Geometry: final body of the model. Coordinates: model frame, mm. Face numbers are marked on the shaded views. Coordinates: 2 decimals unless noted, no trailing zeros. Loops run counter-clockwise (first coordinate to the right, second up) from the corner with the lowest first, then second, coordinate; pieces in that order, holes last. Notation, with made-up numbers: (11.25, 23) - (62.25, 23) arc R24 cw to (62.25, 51) - close; hole circle Ø10 at (34.5, 69). An arc over 180 degrees is marked (long way). Answer in a Markdown table with one row per item.
from build123d import *

# Parameters (mm, degrees)
SKETCH1_R           = 1.3335
SKETCH1_R_2         = 1.5875
BOSS_EXTRUDE1_DEPTH = 1.651
CHAMFER1_SIZE       = 2.54
SKETCH1_2_R         = 1.5875
BOSS_EXTRUDE2_DEPTH = 2.413
SKETCH1_3_R         = 1.5875
CUT_EXTRUDE1_DEPTH  = 0.889
CUT_EXTRUDE2_DEPTH  = 23.382376376


with BuildPart() as part:
    # Sketch1 → Boss-Extrude1 (new body)
    with BuildSketch(Plane(origin=(0, 0, 0), x_dir=(1, 0, 0), z_dir=(0, 1, 0))):
        with BuildLine():
            Line((-5.567119422, 8.9535), (5.567119422, 8.9535))
            ThreePointArc((5.567119422, 8.9535), (6.35, 6.5405), (7.132880578, 8.9535))
            Line((7.132880578, 8.9535), (20.447, 8.9535))
            Line((20.447, 8.9535), (20.447, -8.9535))
            Line((20.447, -8.9535), (7.132880578, -8.9535))
            ThreePointArc((7.132880578, -8.9535), (6.35, -6.5405), (5.567119422, -8.9535))
            Line((5.567119422, -8.9535), (-5.567119422, -8.9535))
            ThreePointArc((-5.567119422, -8.9535), (-6.35, -6.5405), (-7.132880578, -8.9535))
            Line((-7.132880578, -8.9535), (-20.447, -8.9535))
            Line((-20.447, -8.9535), (-20.447, 8.9535))
            Line((-20.447, 8.9535), (-7.132880578, 8.9535))
            ThreePointArc((-7.132880578, 8.9535), (-6.35, 6.5405), (-5.567119422, 8.9535))
        make_face()
        with Locations(Location((-17.8308, 5.6769, 0), (0, 0, 90))):
            Circle(SKETCH1_R, mode=Mode.SUBTRACT)
        with Locations(Location((17.8308, 5.6769, 0), (0, 0, 90))):
            Circle(SKETCH1_R, mode=Mode.SUBTRACT)
        with Locations(Location((17.8308, -5.6769, 0), (0, 0, 90))):
            Circle(SKETCH1_R, mode=Mode.SUBTRACT)
        with Locations(Location((-17.8308, -5.6769, 0), (0, 0, 90))):
            Circle(SKETCH1_R, mode=Mode.SUBTRACT)
        with Locations(Location((-10.414, 5.6769, 0), (0, 0, 90))):
            Circle(SKETCH1_R_2, mode=Mode.SUBTRACT)
        with Locations(Location((10.414, 5.6769, 0), (0, 0, 90))):
            Circle(SKETCH1_R_2, mode=Mode.SUBTRACT)
        with Locations(Location((10.414, -5.6769, 0), (0, 0, 90))):
            Circle(SKETCH1_R_2, mode=Mode.SUBTRACT)
        with Locations(Location((-10.414, -5.6769, 0), (0, 0, 90))):
            Circle(SKETCH1_R_2, mode=Mode.SUBTRACT)
    extrude(amount=BOSS_EXTRUDE1_DEPTH)

    # Chamfer1
    chamfer1_edges = [part.edges().sort_by_distance(p)[0] for p in [
        (20.447, 0.8255, -8.9535),
        (20.447, 0.8255, 8.9535),
        (-20.447, 0.8255, 8.9535),
        (-20.447, 0.8255, -8.9535),
    ]]
    chamfer(chamfer1_edges, length=CHAMFER1_SIZE)

    # Sketch1_2 → Boss-Extrude2 (add)
    with BuildSketch(Plane(origin=(0, 0, 0), x_dir=(1, 0, 0), z_dir=(0, 1, 0))):
        with Locations(Location((-10.414, 5.6769, 0), (0, 0, 270))):
            Circle(SKETCH1_2_R)
        with Locations(Location((10.414, 5.6769, 0), (0, 0, 270))):
            Circle(SKETCH1_2_R)
        with Locations(Location((10.414, -5.6769, 0), (0, 0, 270))):
            Circle(SKETCH1_2_R)
        with Locations(Location((-10.414, -5.6769, 0), (0, 0, 270))):
            Circle(SKETCH1_2_R)
    extrude(amount=BOSS_EXTRUDE2_DEPTH)

    # Sketch1_3 → Cut-Extrude1 (cut)
    with BuildSketch(Plane(origin=(0, 0, 0), x_dir=(1, 0, 0), z_dir=(0, 1, 0))):
        with Locations(Location((-10.414, 5.6769, 0), (0, 0, 270))):
            Circle(SKETCH1_3_R)
        with Locations(Location((10.414, 5.6769, 0), (0, 0, 270))):
            Circle(SKETCH1_3_R)
        with Locations(Location((10.414, -5.6769, 0), (0, 0, 270))):
            Circle(SKETCH1_3_R)
        with Locations(Location((-10.414, -5.6769, 0), (0, 0, 270))):
            Circle(SKETCH1_3_R)
    extrude(amount=CUT_EXTRUDE1_DEPTH, mode=Mode.SUBTRACT)

    # Sketch2 → Cut-Extrude2 (cut, through all)
    with BuildSketch(Plane(origin=(0, 1.651, 0), x_dir=(1, 0, 0), z_dir=(0, 1, 0))):
        with BuildLine():
            Line((-17.907, 1.630758795), (-17.907, -1.630758795))
            Line((-17.907, -1.630758795), (-15.600758795, -3.937))
            Line((-15.600758795, -3.937), (-12.339241205, -3.937))
            Line((-12.339241205, -3.937), (-11.186120602, -2.783879398))
            Line((-11.186120602, -2.783879398), (-10.033, -3.302))
            Line((-10.033, -3.302), (-5.572102386, -3.302))
            ThreePointArc((-5.572102386, -3.302), (0, -6.477), (5.572102386, -3.302))
            Line((5.572102386, -3.302), (10.033, -3.302))
            Line((10.033, -3.302), (11.186120602, -2.783879398))
            Line((11.186120602, -2.783879398), (12.339241205, -3.937))
            Line((12.339241205, -3.937), (15.600758795, -3.937))
            Line((15.600758795, -3.937), (17.907, -1.630758795))
            Line((17.907, -1.630758795), (17.907, 1.630758795))
            Line((17.907, 1.630758795), (15.600758795, 3.937))
            Line((15.600758795, 3.937), (12.339241205, 3.937))
            Line((12.339241205, 3.937), (11.186120602, 2.783879398))
            Line((11.186120602, 2.783879398), (10.033, 3.302))
            Line((10.033, 3.302), (5.572102386, 3.302))
            ThreePointArc((5.572102386, 3.302), (0, 6.477), (-5.572102386, 3.302))
            Line((-5.572102386, 3.302), (-10.033, 3.302))
            Line((-10.033, 3.302), (-11.186120602, 2.783879398))
            Line((-11.186120602, 2.783879398), (-12.339241205, 3.937))
            Line((-12.339241205, 3.937), (-15.600758795, 3.937))
            Line((-15.600758795, 3.937), (-17.907, 1.630758795))
        make_face()
    extrude(amount=-CUT_EXTRUDE2_DEPTH, mode=Mode.SUBTRACT)


solid = part.part
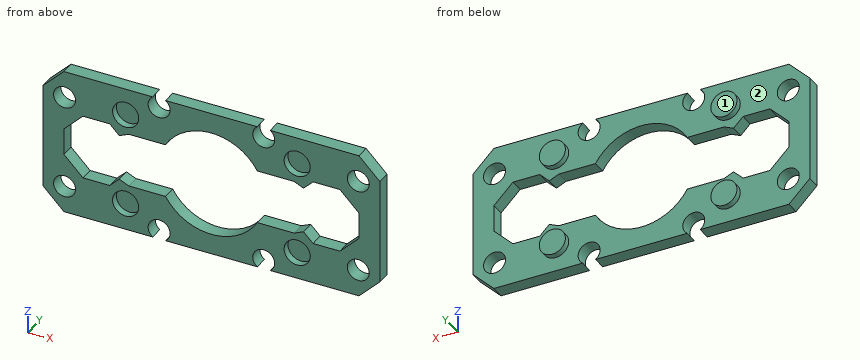
(1) Cut plane C-C on z = -5. State how many separate pieces and enclosed holes the cut face has, then the cut area to 3 significant figures.
Verdict:
| item | result |
|---|---|
| separate pieces | 4 |
| enclosed holes | 0 |
| area | 45.6 mm² |
(2) Cut plane A-A on x = -6.35. Output: boundary loops of the cut face in (y, z), then the cut area to 3 significant figures.
Verdict:
| item | result |
|---|---|
| outline | (0, -6.54) - (1.65, -6.54) - (1.65, -3.3) - (0, -3.3) - close; (0, 3.3) - (1.65, 3.3) - (1.65, 6.54) - (0, 6.54) - close |
| area | 10.7 mm² |
(3) Pull-direction query (X, two-part tool) for the marked faces 1 and 2; classes: pulls with the +X half, pulls with the -X half, needs draft (parallel to the pull), parting line crosses it, or undercut.
Verdict:
| item | result |
|---|---|
| face 1 | needs draft |
| face 2 | undercut |
(4) Cut plane B-B on z = 0. Output: boundary loops of the cut face in (x, y).
Verdict:
| item | result |
|---|---|
| outline | (-20.45, 0) - (-17.91, 0) - (-17.91, 1.65) - (-20.45, 1.65) - close; (17.91, 0) - (20.45, 0) - (20.45, 1.65) - (17.91, 1.65) - close |
(5) Ray query, probe 1 along Z at (x, y) = (-18, 1); probe 2 along X at (y, z) = (0.7, 5); probe 3 along Z at (x, y) = (14, 0.1). Return the intervals inside material, ascending.
Verdict:
| item | result |
|---|---|
| probe 1 | z = -8.86 to -7, -4.35 to 4.35, 7 to 8.86 |
| probe 2 | x = -20.45 to -18.98, -16.68 to -11.85, -8.98 to -4.12, 4.12 to 8.98, 11.85 to 16.68, 18.98 to 20.45 |
| probe 3 | z = -8.95 to -3.94, 3.94 to 8.95 |
(6) First-contact query: pin 1 Ø3 at (x, z) = (13.5, 4.5) entering from +Y; pin 2 Ø2.5 at (x, z) = (6.35, -7.874) entering from -Y; pin 3 Ø3 at (x, z) = (6.35, 7.874) entering from -Y. Flat tips, straight axial feed; report the tip coordinate or a pass-through.
Verdict:
| item | result |
|---|---|
| pin 1 | stops at y = 1.65 |
| pin 2 | passes through |
| pin 3 | stops at y = 0 |
